Check sheet for the modelled part. Datum: model origin and axes. Units: mm. A direction names the side the tool comes from. Round coordinates to 2 decimals unless told otherwise and drop trailing zeros. Loops run counter-clockwise (first coordinate to the right, second up) from the corner with the lowest first, then second, coordinate; pieces in that order, holes last. Notation, with made-up numbers: M 27,-8 L 63,-8 A28 ccw 63,11 Z; hole C -2.5,-16.5 d4. An arc over 180 degrees is marked long. Write item = value, one per line. Start each with the question number.
(1) Scan lines: L1, parallel to Y at x = -2, z = 13; L2, parallel to X at y = 2.4, z = 5; L3, parallel to Z at x = -15.5, y = 2.7. Record each from-to range of solid material in increasing order. Write a range as from..to.
(2) Cross-section at D-D on z = 13.5. Record the boundary of the cut face in (x, y).
(3) Cross-section at A-A on z = 0. Record the boundary of the cut face in (x, y), plus the area to 3 significant figures.
(4) Set-up check for faces 4 (the face through (-5.22, 3.01, -16.84)), 5 (the face through (10.987, 0.986, -0.336)), 6 (the face through (0.389, 2.986, -18.287)): record each of +Z, -Z, +X, -X, +Y, -Y from which the full face is reachable in a straight line by a thin tool's end or side.
(5) Go/stop test with flat-tipped pins: P1, Ø2.5, axis at x = -12.5, z = 0, coming from the -Y side; P2, Ø1, axis at y = 0.5, z = 9, coming from the -X side; P3, Ø6, axis at x = 11, z = -13, coming from the +Y side; P4, Ø4, axis at x = 0, z = -12.5, coming from the +Y side. Record where each tip stops, or that it passes through.
(6) Mould release check, pull along Z, two halves, no side actions. Record for faces 1 (the face through (18.3, 3, -0.1)), 2 (the face through (-15.67, 3.01, -6.04)), 3 (the face through (11, 4, 9)): pulls with the +Z half, pulls with the -Z half, needs draft (parallel to the pull), parting line crosses it, or undercut.
(7) Cross-section at C-C on y = 2.55. Record the boundary of the cut face in (x, z).
(8) Cross-section at B-B on x = -12.5. Record the boundary of the cut face in (y, z), plus the area to 3 significant figures.
from build123d import *

# Parameters (mm, degrees)
EXTRUDE_1_DEPTH     = 4
SKETCH_1_3_R        = 1.55
EXTRUDE_2_DEPTH     = 2
CUT_EXTRUDE_1_DEPTH = 2


with BuildPart() as part:
    # 草图1 → 凸台-拉伸1 (new body)
    with BuildSketch(Plane(origin=(0, 0, 0), x_dir=(1, 0, 0), z_dir=(0, 1, 0))):
        with BuildLine():
            ThreePointArc((6.814196026, 16.295620175), (10.893644329, 10.893644329), (16.295620175, 6.814196026))
            ThreePointArc((16.295620175, 6.814196026), (20.299824853, 0.052271097), (16.386606825, -6.76271302))
            ThreePointArc((16.386606825, -6.76271302), (10.936304212, -10.936304212), (6.76271302, -16.386606825))
            ThreePointArc((6.76271302, -16.386606825), (0, -20.3), (-6.76271302, -16.386606825))
            ThreePointArc((-6.76271302, -16.386606825), (-10.936304212, -10.936304212), (-16.386606825, -6.76271302))
            ThreePointArc((-16.386606825, -6.76271302), (-20.299824853, 0.052271097), (-16.295620175, 6.814196026))
            ThreePointArc((-16.295620175, 6.814196026), (-10.893644329, 10.893644329), (-6.814196026, 16.295620175))
            ThreePointArc((-6.814196026, 16.295620175), (0, 20.3), (6.814196026, 16.295620175))
        make_face()
        with BuildLine():
            ThreePointArc((15.322384233, 5.066966276), (18.299869762, 0.038868252), (15.390040972, -5.02868404))
            ThreePointArc((15.390040972, -5.02868404), (9.52209065, -9.52209065), (5.02868404, -15.390040972))
            ThreePointArc((5.02868404, -15.390040972), (0, -18.3), (-5.02868404, -15.390040972))
            ThreePointArc((-5.02868404, -15.390040972), (-9.52209065, -9.52209065), (-15.390040972, -5.02868404))
            ThreePointArc((-15.390040972, -5.02868404), (-18.299869762, 0.038868252), (-15.322384233, 5.066966276))
            ThreePointArc((-15.322384233, 5.066966276), (-9.479430767, 9.479430767), (-5.066966276, 15.322384233))
            ThreePointArc((-5.066966276, 15.322384233), (0, 18.3), (5.066966276, 15.322384233))
            ThreePointArc((5.066966276, 15.322384233), (9.479430767, 9.479430767), (15.322384233, 5.066966276))
        make_face(mode=Mode.SUBTRACT)
    extrude(amount=EXTRUDE_1_DEPTH)

    # 草图1<3> → 凸台-拉伸2 (add)
    with BuildSketch(Plane(origin=(0, 0, 0), x_dir=(1, 0, 0), z_dir=(0, 1, 0))):
        with BuildLine():
            ThreePointArc((15.390040972, -5.02868404), (9.52209065, -9.52209065), (5.02868404, -15.390040972))
            ThreePointArc((5.02868404, -15.390040972), (0, -18.3), (-5.02868404, -15.390040972))
            ThreePointArc((-5.02868404, -15.390040972), (-9.52209065, -9.52209065), (-15.390040972, -5.02868404))
            ThreePointArc((-15.390040972, -5.02868404), (-18.299869762, 0.038868252), (-15.322384233, 5.066966276))
            ThreePointArc((-15.322384233, 5.066966276), (-9.479430767, 9.479430767), (-5.066966276, 15.322384233))
            ThreePointArc((-5.066966276, 15.322384233), (0, 18.3), (5.066966276, 15.322384233))
            ThreePointArc((5.066966276, 15.322384233), (9.479430767, 9.479430767), (15.322384233, 5.066966276))
            ThreePointArc((15.322384233, 5.066966276), (18.299869762, 0.038868252), (15.390040972, -5.02868404))
        make_face()
        with Locations(Location((0, -12.5, 0), (0, 0, 270))):
            Circle(SKETCH_1_3_R, mode=Mode.SUBTRACT)
        with Locations(Location((12.5, 0, 0), (0, 0, 270))):
            Circle(SKETCH_1_3_R, mode=Mode.SUBTRACT)
        with Locations(Location((0, 12.5, 0), (0, 0, 270))):
            Circle(SKETCH_1_3_R, mode=Mode.SUBTRACT)
        with Locations(Location((-12.5, 0, 0), (0, 0, 270))):
            Circle(SKETCH_1_3_R, mode=Mode.SUBTRACT)
    extrude(amount=EXTRUDE_2_DEPTH)

    # 草图2 → 切除-拉伸1 (cut)
    with BuildSketch(Plane(origin=(0, 4, 0), x_dir=(1, 0, 0), z_dir=(0, 1, 0))):
        Polygon((-17.675489757, 8.235718661), (-13.629873573, 3.804805697), (-2.552591164, 13.918846157), (-6.598207348, 18.349759121), align=None)
    extrude(amount=-CUT_EXTRUDE_1_DEPTH, mode=Mode.SUBTRACT)


solid = part.part
Result:
q1.L1 = 0..2
q1.L2 = -18.49..-15.44, 15.44..18.49
q1.L3 = -5.85..-4.96, 4.96..7.3
q2.outline = M -8.69,0 L -1.18,0 L -1.18,2 L -6.22,2 L -6.22,4 L -8.69,4 Z; M 1.18,0 L 8.69,0 L 8.69,4 L 6.22,4 L 6.22,2 L 1.18,2 Z
q3.outline = M -20.3,0 L -14.05,0 L -14.05,2 L -18.3,2 L -18.3,4 L -20.3,4 Z; M -10.95,0 L 10.95,0 L 10.95,2 L -10.95,2 Z; M 14.05,0 L 20.3,0 L 20.3,4 L 18.3,4 L 18.3,2 L 14.05,2 Z
q3.area = 76.8 mm^2
q4.face_4 = -X, +Y
q4.face_5 = +Y, -Y
q4.face_6 = +Y
q5.P1 = through
q5.P2 = -13.75
q5.P3 = 4
q5.P4 = 2
q6.face_1 = undercut
q6.face_2 = pulls with the -Z half
q6.face_3 = needs draft
q7.outline = M -16.39,6.76 A7.8 ccw -16.35,-6.78 L -14.97,-5.27 A26.5 ccw -15.32,-5.07 A5.8 cw -15.39,5.03 A28.1 ccw -5.03,15.39 A5.8 cw 5.03,15.39 A28.1 ccw 15.39,5.03 A5.8 cw 15.32,-5.07 A26.5 ccw 5.07,-15.32 A5.8 cw -4.55,-16.1 L -5.91,-17.59 A7.8 ccw 6.81,-16.3 A24.5 cw 16.3,-6.81 A7.8 ccw 16.39,6.76 A26.1 cw 6.76,16.39 A7.8 ccw -6.76,16.39 A26.1 cw Z
q8.outline = M 0,-9.42 L 2,-9.42 L 2,-1.55 L 0,-1.55 Z; M 0,1.55 L 2,1.55 L 2,6.94 L 4,6.94 L 4,9.5 L 0,9.5 Z
q8.area = 36.8 mm^2
